Model file for the job. Use its own axes, mm. Face numbers are marked on the shaded views. Give positions to 0.01 mm unless a question says otherwise; leave off trailing zeros. Loops run counter-clockwise (first coordinate to the right, second up) from the corner with the lowest first, then second, coordinate; pieces in that order, holes last. Notation, with made-up numbers: (20, 7.25) -> (51, 7.25) arc R25 ccw to (51, 44.25) -> close; hole circle Ø8 at (12.25, 40). An arc over 180 degrees is marked (long way). Use CSV: the item, a comma, the result in double quotes. Start each with the question number.
(1) Flat gauge pins, fed straight in: pin 1 (5 mm diameter, centred on y = -112.4, z = -6.3, fed in from +X); pin 2 (3 mm diameter, centred on x = 5.5, y = 17.5, fed in from +Z). Where does each tip first touch, or does it go through?
(2) Cut at B-B on z = 6.3. State how many separate pieces and enclosed holes the cut face has, then the cut area to 3 significant figures.
(3) Drill centre lines: probe 1 along Y at (x, z) = (2.6, -6.3) (3 decimals); probe 2 along Z at (x, y) = (9.5, 18); probe 3 along Y at (x, z) = (4.5, 0). Where is each one in solid material? Low to high.
(4) Pull direction Y, two halves, no side cores. Call the marked faces 1, 2, 3 and 4: pulls with the +Y half, pulls with the -Y half, needs draft (parallel to the pull), parting line crosses it, or undercut.
(5) Cut at A-A on y = 0. Write the cut outline in (x, z), then the cut area to 3 significant figures.
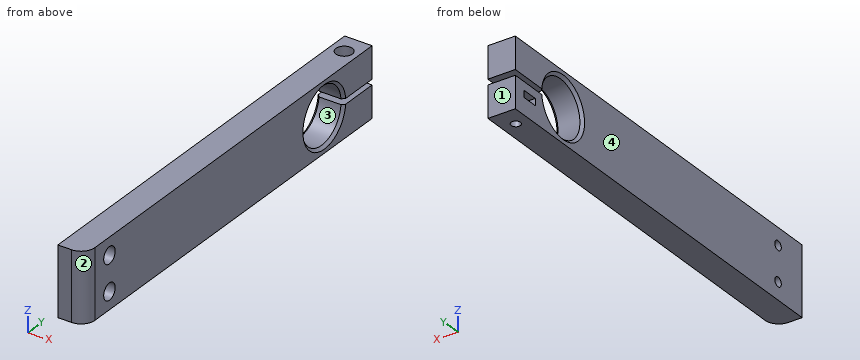
from build123d import *

# Parameters (mm, degrees)
SKETCH1_R           = 10.2
BOSS_EXTRUDE1_DEPTH = 10
SKETCH2_R           = 1.7
CUT_EXTRUDE2_DEPTH  = 127.030789889
SKETCH5_W           = 2
SKETCH5_H           = 25
CUT_EXTRUDE4_DEPTH  = 127.030789889
SKETCH7_R           = 1.7
CUT_EXTRUDE5_DEPTH  = 128.906372007
CUT_EXTRUDE7_DEPTH  = 2.5
FILLET1_R           = 5
CHAMFER1_SIZE       = 1
SKETCH9_R           = 3
CUT_EXTRUDE8_DEPTH  = 8
SKETCH13_R          = 3
CUT_EXTRUDE9_DEPTH  = 5


with BuildPart() as part:
    # Sketch1 → Boss-Extrude1 (new body)
    with BuildSketch(Plane(origin=(0, 0, 0), x_dir=(0, 0, -1), z_dir=(1, 0, 0))):
        Polygon((-12.6, -25), (-12.6, -125), (12.6, -125), (12.6, -25), (12.6, 25), (-12.6, 25), align=None)
        Circle(SKETCH1_R, mode=Mode.SUBTRACT)
    extrude(amount=BOSS_EXTRUDE1_DEPTH)

    # Sketch2 → Cut-Extrude2 (cut, through all)
    with BuildSketch(Plane(origin=(0, 0, 0), x_dir=(0, 0, -1), z_dir=(1, 0, 0))):
        with Locations((-6.3, -112.4)):
            Circle(SKETCH2_R)
        with Locations((6.3, -112.4)):
            Circle(SKETCH2_R)
    extrude(amount=CUT_EXTRUDE2_DEPTH, mode=Mode.SUBTRACT)

    # Sketch5 → Cut-Extrude4 (cut, through all)
    with BuildSketch(Plane.ZY):
        with Locations((0, 12.5)):
            Rectangle(SKETCH5_W, SKETCH5_H)
    extrude(amount=-CUT_EXTRUDE4_DEPTH, mode=Mode.SUBTRACT)

    # Sketch7 → Cut-Extrude5 (cut, through all)
    with BuildSketch(Plane.XY.offset(12.6)):
        with Locations((5, 17.575)):
            Circle(SKETCH7_R)
    extrude(amount=-CUT_EXTRUDE5_DEPTH, mode=Mode.SUBTRACT)

    # Sketch8 → Cut-Extrude7 (cut)
    with BuildSketch(Plane.XY.offset(-4)):
        Polygon((3.267949192, 20.575), (0, 20.575), (0, 14.575), (3.267949192, 14.575), (6.732050808, 14.575), (8.464101615, 17.575), (6.732050808, 20.575), align=None)
    extrude(amount=-CUT_EXTRUDE7_DEPTH, mode=Mode.SUBTRACT)

    # Fillet1
    fillet1_edges = [part.edges().sort_by_distance(p)[0] for p in [
        (10, -125, 0),
    ]]
    fillet(fillet1_edges, radius=FILLET1_R)

    # Chamfer1
    chamfer1_edges = [part.edges().sort_by_distance(p)[0] for p in [
        (10, -10.2, 0),
        (0, -10.2, 0),
    ]]
    chamfer(chamfer1_edges, length=CHAMFER1_SIZE)

    # Sketch9 → Cut-Extrude8 (cut)
    with BuildSketch(Plane.XY.offset(12.6)):
        with Locations((5, 17.575)):
            Circle(SKETCH9_R)
    extrude(amount=-CUT_EXTRUDE8_DEPTH, mode=Mode.SUBTRACT)

    # Sketch13 → Cut-Extrude9 (cut)
    with BuildSketch(Plane(origin=(10, 0, 0), x_dir=(0, 0, -1), z_dir=(1, 0, 0))):
        with Locations((6.3, -112.4)):
            Circle(SKETCH13_R)
        with Locations((-6.3, -112.4)):
            Circle(SKETCH13_R)
    extrude(amount=-CUT_EXTRUDE9_DEPTH, mode=Mode.SUBTRACT)


solid = part.part
Check result:
1,pin 1,"x = 5"
1,pin 2,"z = 4.6"
2,separate pieces,"3"
2,enclosed holes,"1"
2,area,"1,260 mm²"
3,probe 1,"-125 to -114.1, -110.7 to -8.022, 8.022 to 14.575, 20.575 to 25"
3,probe 2,"-12.6 to -1, 1 to 12.6"
3,probe 3,"-125 to -10.2"
4,face 1,"pulls with the +Y half"
4,face 2,"pulls with the -Y half"
4,face 3,"undercut"
4,face 4,"needs draft"
5,outline,"(0, -12.6) -> (10, -12.6) -> (10, -11.2) -> (9, -10.2) -> (1, -10.2) -> (0, -11.2) -> close; (0, 11.2) -> (1, 10.2) -> (9, 10.2) -> (10, 11.2) -> (10, 12.6) -> (0, 12.6) -> close"
5,area,"46.0 mm²"
